Autodesk Inventor part; units mm, degrees
ref_plane "YZ Plane" through (0, 0, 0) normal (1, 0, 0) x (0, 1, 0)
ref_plane "XZ Plane" through (0, 0, 0) normal (0, 1, 0) x (-1, 0, 0)
ref_plane "XY Plane" through (0, 0, 0) normal (0, 0, 1) x (1, 0, 0)
sketch "Esboço1" plane through (0, 0, 0) normal (0, 0, 1) x (1, 0, 0)
  circle A0 centre (0, 0) radius 8
  dimension "d0" = 16
extrude "Extrusão1" add sketch "Esboço1" along normal mid plane 320
sketch "Esboço2" plane through (0, 0, 0) normal (1, 0, 0) x (0, 1, 0)
  line L0 (8, -160) -> (8, 160)
  line L1 (8, -135) -> (6.5, -135)
  line L2 (6.5, -135) -> (6.5, -137)
  line L3 (6.5, -137) -> (8, -137)
  line L4 (8, -137) -> (8, -135)
  line L5 (8, 137) -> (6.5, 137)
  line L6 (6.5, 137) -> (6.5, 135)
  line L7 (6.5, 135) -> (8, 135)
  line L8 (8, 135) -> (8, 137)
  line L9 (8, 160) -> (-8, 160)
  line L10 (-8, -160) -> (8, -160)
  line L11 (0, 0) -> (0, -160)
  dimension "d3" = 2
  dimension "d4" = 25
  dimension "d5" = 2
  dimension "d6" = 25
  dimension "d7" = 13
revolve "Revolução1" cut sketch "Esboço2" angle 360 about axis through (0, 0, 0) along (0, 0, -1)
thread "Rosca1"
chamfer "Chanfro1" distance 1.5 angle 45 2 edges at (-8, 0, 160) (-8, 0, -160)
Build history of the part. All positions in model axes, mm. A direction names the side the tool comes from. Round coordinates to 2 decimals unless told otherwise and drop trailing zeros. Write each loop counter-clockwise with the first axis right and the second up, starting at its lowest first coordinate (ties: lowest second). Pieces come first, ordered by that corner, then holes. Notation, with made-up numbers: (37, 64.25) - (44, 64.25) arc R23 cw to (44, 92.25) - close; hole circle Ø10 at (67, 52.25). An arc over 180 degrees is marked (long way). Use CSV: the item, a comma, the result in double quotes.
(1) 3-axis set-ups, long thin cutter, end or side, ignore diameter. For faces 5 (the cylindrical face through (-1.73, -7.81, -147.6)), 6 (the cylindrical face through (-3.955, -5.158, 135.986)): which of +Z, -Z, +X, -X, +Y, -Y reach the whole face in a straight line?
Response:
face 5,"+Z, -Z"
face 6,"none"
(2) Pin check, flat tips, straight feed: P1, Ø1, axis at y = -5, z = -1.5, coming from the -X side; P2, Ø1, axis at y = -5, z = 112, coming from the +X side; P3, Ø6, axis at x = 6, z = -84, coming from the +Y side. Stop position of each tip, or through.
Response:
P1,"x = -6.61"
P2,"x = 6.61"
P3,"y = 7.42"
(3) Band-saw the part on A-A (z = -96). Write the cut outline in (x, y), plus the area to 3 significant figures.
Response:
outline,"circle Ø16 at (0, 0)"
area,"201 mm²"
(4) Wall check: line 1 (Z direction, x = -1.75, y = 6.75); line 2 (Z direction, x = -3.25, y = -6.5); line 3 (Y direction, x = -4.75, z = -110). Give the ranges that are in metal, low to high.
Response:
line 1,"-159.53 to -137, -135 to 135, 137 to 159.53"
line 2,"-159.23 to -137, -135 to 135, 137 to 159.23"
line 3,"-6.44 to 6.44"
(5) Mould opens along Z. For faces 1 (the flat face through (7, 0, 135)), 2 (the cylindrical face through (-1.73, 7.81, -1.89)), 3 (the flat face through (7, 0, -135)), 4 (the flat face through (0, 0, 160)) say: pulls with the +Z half, pulls with the -Z half, needs draft (parallel to the pull), parting line crosses it, or undercut.
Response:
face 1,"undercut"
face 2,"needs draft"
face 3,"undercut"
face 4,"pulls with the +Z half"
